Could you check a few things on this model? Use its own coordinates, in mm. Face numbers are marked on the shaded views. A direction names the side the tool comes from. Coordinates: 2 decimals unless noted, no trailing zeros. Loops run counter-clockwise (first coordinate to the right, second up) from the corner with the lowest first, then second, coordinate; pieces in that order, holes last. Notation, with made-up numbers: (47, 43.5) - (77, 43.5) arc R21 ccw to (77, 65.5) - close; hole circle Ø6 at (85, 49). An arc over 180 degrees is marked (long way). Use CSV: the item, a comma, the result in double quotes.
from build123d import *

# Parameters (mm, degrees)
SKETCH1_W           = 33
SKETCH1_H           = 23
BOSS_EXTRUDE1_DEPTH = 5
SKETCH2_W           = 21
SKETCH2_H           = 10
BOSS_EXTRUDE2_DEPTH = 27
FILLET1_R           = 1
SKETCH3_R           = 1.15
BOSS_EXTRUDE5_DEPTH = 2.8
FILLET9_R           = 0.25


with BuildPart() as part:
    # Sketch1 → Boss-Extrude1 (new body)
    with BuildSketch(Plane(origin=(0, 0, 0), x_dir=(0, 0, -1), z_dir=(1, 0, 0))):
        with Locations((16.5, 11.5)):
            Rectangle(SKETCH1_W, SKETCH1_H)
    extrude(amount=BOSS_EXTRUDE1_DEPTH)

    # Sketch2 → Boss-Extrude2 (add)
    with BuildSketch(Plane.ZY):
        with Locations((-16.5, 11.5)):
            Rectangle(SKETCH2_W, SKETCH2_H)
    extrude(amount=BOSS_EXTRUDE2_DEPTH)

    # Fillet1
    fillet1_edges = [part.edges().sort_by_distance(p)[0] for p in [
        (-27, 11.5, -27),
        (-27, 6.5, -16.5),
        (-27, 11.5, -6),
        (-27, 16.5, -16.5),
    ]]
    fillet(fillet1_edges, radius=FILLET1_R)

    # Sketch3 → Boss-Extrude5 (add)
    with BuildSketch(Plane.ZY):
        with Locations((-2.25, 11.5)):
            Circle(SKETCH3_R)
        with Locations((-30.75, 11.5)):
            Circle(SKETCH3_R)
    extrude(amount=BOSS_EXTRUDE5_DEPTH)

    # Fillet9
    fillet9_edges = [part.edges().sort_by_distance(p)[0] for p in [
        (0, 11.5, -3.4),
        (0, 11.5, -31.9),
    ]]
    fillet(fillet9_edges, radius=FILLET9_R)


solid = part.part
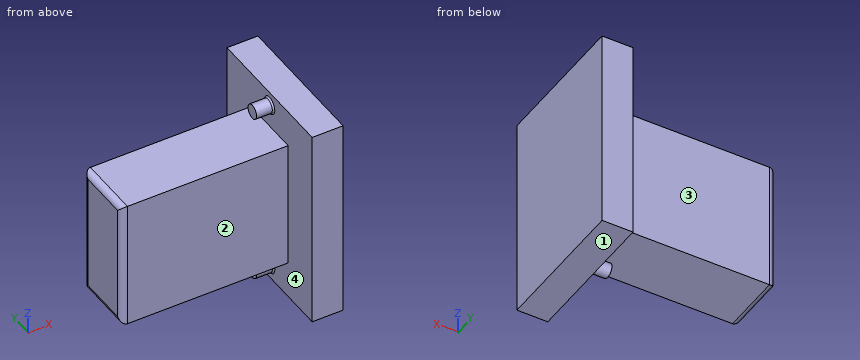
(1) Please list where these lines run through material, in increasing order: line 1 (Y direction, x = -6, z = -14); line 2 (X direction, y = 1.75, z = -18.5); line 3 (Z direction, x = -13, y = 13.5).
Computed:
line 1,"y = 6.5 to 16.5"
line 2,"x = 0 to 5"
line 3,"z = -27 to -6"
(2) Which directions (+Z, -Z, +X, -X, +Y, -Y) give clear straight access to the entire face, cutting with the end or side of a thin tool? Please do the marked faces 1, 2, 3 and 4.
Computed:
face 1,"-Z, +X, -X, +Y, -Y"
face 2,"+Z, -Z, -X, -Y"
face 3,"+Z, -Z, -X, +Y"
face 4,"-X"
(3) Will these pins go through, and if not, where does the flat tip stop? pin 1 (3 mm diameter, centred on x = -0.5, z = -27, fed in from -Y); pin 2 (2 mm diameter, centred on y = 20, z = -18.5, fed in from -X); pin 3 (1.1 mm diameter, centred on y = 11.5, z = -31, fed in from -X); pin 4 (6 mm diameter, centred on x = -12, y = 2.5, fed in from -Z).
Computed:
pin 1,"stops at y = 0"
pin 2,"stops at x = 0"
pin 3,"stops at x = -2.8"
pin 4,"passes through"
(4) Suppose I cut it at A-A (z = -2.25). Write out the boundary of the cut face in (x, y), plus the area to 3 significant figures.
Computed:
outline,"(-2.8, 10.35) - (-0.25, 10.35) arc R0.25 cw to (0, 10.1) - (0, 0) - (5, 0) - (5, 23) - (0, 23) - (0, 12.9) arc R0.25 cw to (-0.25, 12.65) - (-2.8, 12.65) - close"
area,"121 mm²"
(5) Suppose I cut it at C-C (x = -14.5). Write out the boundary of the cut face in (y, z), plus the area to 3 significant figures.
Computed:
outline,"(6.5, -27) - (16.5, -27) - (16.5, -6) - (6.5, -6) - close"
area,"210 mm²"
(6) Suppose I cut it at B-B (y = 8.25). Write out the boundary of the cut face in (x, z).
Computed:
outline,"(-27, -26) arc R1 ccw to (-26, -27) - (0, -27) - (0, -33) - (5, -33) - (5, 0) - (0, 0) - (0, -6) - (-26, -6) arc R1 ccw to (-27, -7) - close"
